```python
from build123d import *

# Parameters (mm, degrees)
SKETCH1_W           = 165
SKETCH1_H           = 240
BOSS_EXTRUDE1_DEPTH = 3
SKETCH3_R           = 1.6
CUT_EXTRUDE2_DEPTH  = 11
SKETCH2_W           = 18
SKETCH2_H           = 38
CUT_EXTRUDE1_DEPTH  = 11
FILLET1_R           = 5


with BuildPart() as part:
    # Sketch1 → Boss-Extrude1 (new body)
    with BuildSketch(Plane(origin=(0, 0, 0), x_dir=(1, 0, 0), z_dir=(0, 1, 0))):
        Rectangle(SKETCH1_W, SKETCH1_H)
    extrude(amount=BOSS_EXTRUDE1_DEPTH)

    # Sketch3 → Cut-Extrude2 (cut)
    with BuildSketch(Plane(origin=(0, 3, 0), x_dir=(1, 0, 0), z_dir=(0, 1, 0))):
        with Locations((15, 46)):
            Circle(SKETCH3_R)
        with Locations((-15, 46)):
            Circle(SKETCH3_R)
        with Locations((15, -4)):
            Circle(SKETCH3_R)
        with Locations((-15, -4)):
            Circle(SKETCH3_R)
        with Locations((15, -54)):
            Circle(SKETCH3_R)
        with Locations((-15, -54)):
            Circle(SKETCH3_R)
        with Locations((15, -104)):
            Circle(SKETCH3_R)
        with Locations((-15, -104)):
            Circle(SKETCH3_R)
    extrude(amount=-CUT_EXTRUDE2_DEPTH, mode=Mode.SUBTRACT)

    # Sketch2 → Cut-Extrude1 (cut)
    with BuildSketch(Plane(origin=(0, 3, 0), x_dir=(1, 0, 0), z_dir=(0, 1, 0))):
        with Locations((73.5, 101)):
            Rectangle(SKETCH2_W, SKETCH2_H)
        with Locations((73.5, -101)):
            Rectangle(SKETCH2_W, SKETCH2_H)
    extrude(amount=-CUT_EXTRUDE1_DEPTH, mode=Mode.SUBTRACT)

    # Fillet1
    fillet1_edges = [part.edges().sort_by_distance(p)[0] for p in [
        (64.5, 1.5, -82),
        (64.5, 1.5, 82),
    ]]
    fillet(fillet1_edges, radius=FILLET1_R)


solid = part.part
```
Input: part model. Units: mm. Frame: model coordinates. Give positions to 0.01 mm unless a question says otherwise; leave off trailing zeros. Order: outer loops, then holes, each group sorted by start corner. A loop starts at its lowest first (then second) coordinate and runs counter-clockwise, first axis right, second up. Notation, with made-up numbers: (63.5, 82) -> (122.5, 82) arc R15 cw to (122.5, 90) -> close; hole circle Ø5 at (84.25, -34). An arc over 180 degrees is marked (long way). Write each question's results on one line, items separated by ' | '. Start each with the question number.
Item 1: Cut plane A-A on y = 0.55. Give the number of separate pieces and of enclosed holes in the cut face, then the cut area to 3 significant figures.
Item 2: Contact query for flat-ended pins moving along their axis: P1, Ø0.9, axis at y = 1, z = 97.5, coming from the +X side; P2, Ø5, axis at x = 15, z = -46, coming from the -Y side; P3, Ø3, axis at x = -15, z = 104, coming from the +Y side. Output: stop coordinate, or through.
Item 3: Cut plane B-B on z = -97.5. Return the cut outline in (x, y).
Item 4: Line query: line 1 (X direction, y = 1.55, z = 54); line 2 (X direction, y = 2.2, z = 104); line 3 (Z direction, x = -15, y = 1.05). Output: solid intervals per line, ascending.
Established:
1) separate pieces: 1 | enclosed holes: 8 | area: 38,200 mm^2
2) P1: x = 64.5 | P2: y = 0 | P3: through
3) outline: (-82.5, 0) -> (64.5, 0) -> (64.5, 3) -> (-82.5, 3) -> close
4) line 1: -82.5 to -16.6, -13.4 to 13.4, 16.6 to 82.5 | line 2: -82.5 to -16.6, -13.4 to 13.4, 16.6 to 64.5 | line 3: -120 to -47.6, -44.4 to 2.4, 5.6 to 52.4, 55.6 to 102.4, 105.6 to 120
